from build123d import *

# Parameters (mm, degrees)
F0_R     = 15
F1_DEPTH = 150
F2_T     = -2.5
F5_W     = 16
F5_H     = 30
F6_DEPTH = 220
F7_R     = 5.38096
F8_DEPTH = 200


with BuildPart() as f1:
    # F0 (on Top) → F1 (new body)
    with BuildSketch(Plane.XY):
        Circle(F0_R)
    extrude(amount=F1_DEPTH)

    # F2
    f2_openings = [f1.faces().sort_by_distance(p)[0] for p in [
        (0, 0, 150),
    ]]
    offset(amount=F2_T, openings=f2_openings)

    # F5 (on face) → F6 (join)
    with BuildSketch(Plane(origin=(0, 0, 0), x_dir=(0, -1, 0), z_dir=(-0.707107, 0, 0.707107))):
        with Locations((2.385001, -3.465989)):
            Rectangle(F5_W, F5_H)
    extrude(amount=F6_DEPTH)

    # F7 (on Right) → F8 (join)
    with BuildSketch(Plane.YZ):
        with Locations((0, 140.51652)):
            Circle(F7_R)
    extrude(amount=-F8_DEPTH)


solid = f1.part
Geometry: final body of the model. Coordinates: model frame, mm. A direction names the side the tool comes from. Give positions to 0.01 mm unless a question says otherwise; leave off trailing zeros. Loops run counter-clockwise (first coordinate to the right, second up) from the corner with the lowest first, then second, coordinate; pieces in that order, holes last. Notation, with made-up numbers: M 4,11.5 L 10,11.5 A30 ccw 10,46.5 Z; hole C -4,-12 d5. An arc over 180 degrees is marked long. Put each result on its own line as item: value. Start each with the question number.
1) Ray query, line 1 along Y through (x, z) = (0, 75); line 2 along X through (y, z) = (0, 47.5); line 3 along X through (y, z) = (0, 44). Return the intervals inside material, ascending.
2) Pull-direction query (Z, two-part tool) for faces 1 (the flat face through (-2.03, -2.27, 18.34)), 2 (the flat face through (-78.16, -2.27, 94.47)), 3 (the flat face through (-157.866, -2.273, 153.261)), 4 (the flat face through (-200, 0, 141)); classes: pulls with the +Z half, pulls with the -Z half, needs draft (parallel to the pull), parting line crosses it, or undercut.
3) Cut plane B-B (y = 2.5). Output: boundary loops of the cut face in (x, z).
4) Cut plane C-C (x = -118). Output: boundary loops of the cut face in (y, z) (3 decimals).
5) Cut plane A-A (z = 37). Output: boundary loops of the cut face in (x, y) (3 decimals).
6) Contact query for flat-ended pins moving along their axis: pin 1 (10 mm diameter, centred on x = -123, y = 5, fed in from -Z); pin 2 (1.5 mm diameter, centred on y = 7, z = 45, fed in from -X); pin 3 (12 mm diameter, centred on x = -4, y = 4, fed in from +Z). Output: stop coordinate, or through.
7) Access query for faces 5 (the flat face through (0, 0, 141)), 6 (the flat face through (-3.4, 12.3, 150)), 7 (the flat face through (5, -2, 5)). Directions: +Z, -Z, +X, -X, +Y, -Y. A direction counts if a zero-diameter tool reaches every point of the face in a straight line with its end or side. Return the directions, or none.
Verdict:
1. line 1: -15 to -12.5, 12.5 to 15
1. line 2: -73.61 to -31.19, -15 to -12.5, 12.5 to 15
1. line 3: -70.11 to -27.69, -15 to -12.5, 12.5 to 15
2. face 1: undercut
2. face 2: undercut
2. face 3: pulls with the +Z half
2. face 4: needs draft
3. outline: M -200,135.75 L -161.87,135.75 L -13.06,-13.06 L 0,0 L 14.79,0 L 14.79,150 L 12.25,150 L 12.25,2.5 L 2.5,2.5 L 8.16,8.16 L -12.25,28.56 L -12.25,135.75 L 0,135.75 L 0,145.28 L -12.25,145.28 L -12.25,150 L -14.79,150 L -14.79,145.28 L -128.97,145.28 L -147.41,163.72 L -165.85,145.28 L -200,145.28 Z; hole M -119.44,135.75 L -14.79,31.1 L -14.79,135.75 Z
4. outline: M -10.385,91.885 L 5.615,91.885 L 5.615,134.312 L -10.385,134.312 Z; C 0,140.517 d10.762
5. outline: M -63.115,-10.385 L -20.688,-10.385 L -20.688,5.615 L -63.115,5.615 Z; C 0,0 d30; hole C 0,0 d25
6. pin 1: z = 91.89
6. pin 2: x = -13.64
6. pin 3: z = 145.9
7. face 5: +Z
7. face 6: +Z, +X, +Y, -Y
7. face 7: none
